```python
from build123d import *

# Parameters (mm, degrees)
CROQUIS1_R                       = 32.7
CROQUIS1_R_2                     = 21
SALIENTE_EXTRUIR1_DEPTH          = 23.5
CROQUIS3_R                       = 32.7
SALIENTE_EXTRUIR3_DEPTH          = 5
CROQUIS4_R                       = 3.5
CORTAR_EXTRUIR1_DEPTH            = 6
CROQUIS21_R                      = 30
SALIENTE_EXTRUIR4_DEPTH          = 10
TALADRO_DE_MARGEN_PARA_M31_D     = 3.4
TALADRO_DE_MARGEN_PARA_M31_DEPTH = 10
TALADRO_DE_MARGEN_PARA_M31_TIP   = 1.021463052


with BuildPart() as part:
    # Croquis1 → Saliente-Extruir1 (new, symmetric)
    with BuildSketch(Plane(origin=(0, 0, 0), x_dir=(0, 0, -1), z_dir=(1, 0, 0))):
        Circle(CROQUIS1_R)
        Circle(CROQUIS1_R_2, mode=Mode.SUBTRACT)
    extrude(amount=SALIENTE_EXTRUIR1_DEPTH, both=True)

    # Croquis3 → Saliente-Extruir3 (add)
    with BuildSketch(Plane.ZY.offset(23.5)):
        Circle(CROQUIS3_R)
        with BuildLine():
            Line((-18, 21), (18, 21))
            ThreePointArc((18, 21), (20.121320344, 20.121320344), (21, 18))
            Line((21, 18), (21, -18))
            ThreePointArc((21, -18), (20.121320344, -20.121320344), (18, -21))
            Line((18, -21), (-18, -21))
            ThreePointArc((-18, -21), (-20.121320344, -20.121320344), (-21, -18))
            Line((-21, -18), (-21, 18))
            ThreePointArc((-21, 18), (-20.121320344, 20.121320344), (-18, 21))
        make_face(mode=Mode.SUBTRACT)
    extrude(amount=SALIENTE_EXTRUIR3_DEPTH)

    # Croquis4 → Cortar-Extruir1 (cut)
    with BuildSketch(Plane.ZY.offset(23.5)):
        with Locations((15.5, 15.5)):
            Circle(CROQUIS4_R)
        with Locations((-15.5, 15.5)):
            Circle(CROQUIS4_R)
        with Locations((-15.5, -15.5)):
            Circle(CROQUIS4_R)
        with Locations((15.5, -15.5)):
            Circle(CROQUIS4_R)
    extrude(amount=-CORTAR_EXTRUIR1_DEPTH, mode=Mode.SUBTRACT)

    # Croquis21 → Saliente-Extruir4 (add)
    with BuildSketch(Plane.ZY.offset(28.5)):
        Circle(CROQUIS21_R)
        with BuildLine():
            Line((18, 21), (0, 21))
            Line((0, 21), (-18, 21))
            ThreePointArc((-18, 21), (-20.121320344, 20.121320344), (-21, 18))
            Line((-21, 18), (-21, 0))
            Line((-21, 0), (-21, -18))
            ThreePointArc((-21, -18), (-20.121320344, -20.121320344), (-18, -21))
            Line((-18, -21), (0, -21))
            Line((0, -21), (18, -21))
            ThreePointArc((18, -21), (20.121320344, -20.121320344), (21, -18))
            Line((21, -18), (21, 0))
            Line((21, 0), (21, 18))
            ThreePointArc((21, 18), (20.121320344, 20.121320344), (18, 21))
        make_face(mode=Mode.SUBTRACT)
    extrude(amount=SALIENTE_EXTRUIR4_DEPTH)

    # Taladro de margen para M31
    with Locations(Plane(origin=(23.5, 0, 0), x_dir=(0, 0, -1), z_dir=(1, 0, 0))):
        with Locations((29, 0), (14.5, -25.11473671), (-14.5, -25.11473671), (-29, 0), (-14.5, 25.11473671), (14.5, 25.11473671)):
            Hole(TALADRO_DE_MARGEN_PARA_M31_D / 2, depth=TALADRO_DE_MARGEN_PARA_M31_DEPTH)
            with Locations((0, 0, -(TALADRO_DE_MARGEN_PARA_M31_DEPTH + TALADRO_DE_MARGEN_PARA_M31_TIP / 2))):  # 118° drill point
                Cone(0, TALADRO_DE_MARGEN_PARA_M31_D / 2, TALADRO_DE_MARGEN_PARA_M31_TIP, mode=Mode.SUBTRACT)


solid = part.part
```
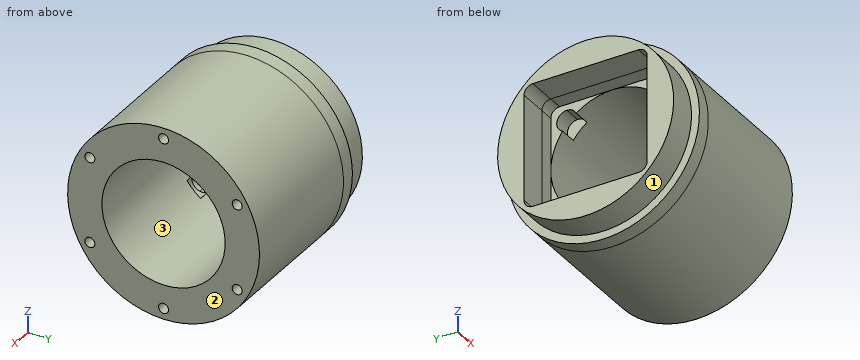
For this review, take the finished solid that the model builds, in its own axes (mm). Face numbers are marked on the shaded views. Round coordinates to 2 decimals unless told otherwise and drop trailing zeros. Write each loop counter-clockwise with the first axis right and the second up, starting at its lowest first coordinate (ties: lowest second). Pieces come first, ordered by that corner, then holes. Notation, with made-up numbers: (-38.5, -29) -> (-21.5, -29) arc R25 cw to (-21.5, -3) -> close; hole circle Ø6 at (51.25, 61). An arc over 180 degrees is marked (long way). Use one line per item in the form item = value.
Q1. Consider section A-A (y = 7). State the section outline as (x, z) points, then the cut area to 3 significant figures.
Resolved:
outline = (-38.5, -29.17) -> (-28.5, -29.17) -> (-28.5, -31.94) -> (23.5, -31.94) -> (23.5, -19.8) -> (-23.5, -19.8) -> (-23.5, -21) -> (-38.5, -21) -> close; (-38.5, 21) -> (-23.5, 21) -> (-23.5, 19.8) -> (23.5, 19.8) -> (23.5, 31.94) -> (-28.5, 31.94) -> (-28.5, 29.17) -> (-38.5, 29.17) -> close
area = 1,410 mm²
Q2. Consider section C-C (x = -19.5). State the section outline as (y, z) points.
Resolved:
outline = circle Ø65.4 at (0, 0); hole (-17, -12.34) arc R3.5 ccw (long way) to (-12.34, -17) arc R21 ccw to (12.34, -17) arc R3.5 ccw (long way) to (17, -12.34) arc R21 ccw to (17, 12.34) arc R3.5 ccw (long way) to (12.34, 17) arc R21 ccw to (-12.34, 17) arc R3.5 ccw (long way) to (-17, 12.34) arc R21 ccw to start
Q3. Consider section D-D (x = 18). State the section outline as (y, z) points, then the cut area to 3 significant figures.
Resolved:
outline = circle Ø65.4 at (0, 0); hole circle Ø3.4 at (-25.11, -14.5); hole circle Ø3.4 at (-25.11, 14.5); hole circle Ø42 at (0, 0); hole circle Ø3.4 at (0, -29); hole circle Ø3.4 at (0, 29); hole circle Ø3.4 at (25.11, -14.5); hole circle Ø3.4 at (25.11, 14.5)
area = 1,920 mm²
Q4. The part is to be moulded in two halves that separate along Y. For the marked faces 1, 2 and 3, say which applies: released by +Y, released by -Y, zero draft, split by the parting line, or undercut.
Resolved:
face_1 = split by the parting line
face_2 = zero draft
face_3 = undercut
Q5. Clearance check with flat-ended pins moving along their axes: pin 1 Ø4 at (x, y) = (-25, 5.5) entering from -Z; pin 2 Ø3 at (x, z) = (15, -3) entering from -Y; pin 3 Ø1 at (x, z) = (-5, -10.5) entering from -Y; pin 4 Ø8 at (x, y) = (2, -2.5) entering from +Z. State where each tip first meets the part, or that it passes through.
Resolved:
pin_1 = -32.51
pin_2 = -32.67
pin_3 = -31.13
pin_4 = 32.7
Q6. To check wall thickness, follow probe 1 along Y at (x, z) = (-36, -0.5); probe 2 along Z at (x, y) = (-3, 0); probe 3 along Y at (x, z) = (21.5, -14.5). State the ranges of each line that lie inside material, in increasing order. Write a range as from..to.
Resolved:
probe_1 = -30..-21, 21..30
probe_2 = -32.7..-21, 21..32.7
probe_3 = -29.31..-26.81, -23.41..-15.19, 15.19..23.41, 26.81..29.31
Q7. Consider section B-B (z = -2). State the section outline as (x, y) points.
Resolved:
outline = (-38.5, -29.93) -> (-28.5, -29.93) -> (-28.5, -32.64) -> (23.5, -32.64) -> (23.5, -20.9) -> (-23.5, -20.9) -> (-23.5, -21) -> (-38.5, -21) -> close; (-38.5, 21) -> (-23.5, 21) -> (-23.5, 20.9) -> (23.5, 20.9) -> (23.5, 32.64) -> (-28.5, 32.64) -> (-28.5, 29.93) -> (-38.5, 29.93) -> close
